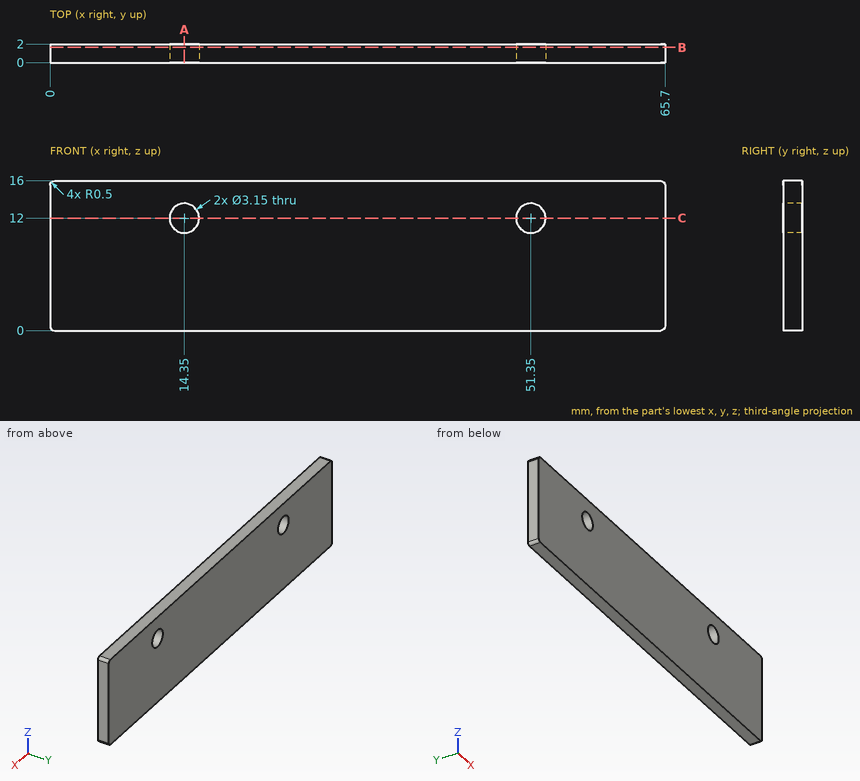
Can you work these out from the drawing? Everything is in mm from the part's minimum corner. Give positions to 0.01 mm unless a question says otherwise; leave off trailing zeros. Loops run counter-clockwise (first coordinate to the right, second up) from the corner with the lowest first, then second, coordinate; pieces in that order, holes last. Notation, with made-up numbers: M 8,-37.5 L 34,-37.5 A28 ccw 34,-8.5 Z; hole C -6.75,-6.5 d11. An arc over 180 degrees is marked long. Use CSV: the item, a comma, the result in double quotes. Start each with the question number.
1. If I drill on L1, parallel to X at y = 1.25, z = 12 (3 decimals); L2, parallel to Z at x = 51.35, y = 0.95 (3 decimals); L3, parallel to Z at x = 51, y = 0.1, over which ranges is the centre line in solid material (lowest first)?
2. Imagine slicing it at A-A, the plane x = 14.35. Write out the boundary of the cut face in (y, z) (3 decimals), plus the area to 3 significant figures.
3. Imagine slicing it at C-C, the plane z = 12. Write out the boundary of the cut face in (x, y) (3 decimals), plus the area to 3 significant figures.
4. For P1, Ø1.9, axis at x = 51.35, z = 12, coming from the +Y side, with a flat end and sliding along its axis, tell me the tip position at first contact or that it passes through.
5. Imagine slicing it at B-B, the plane y = 1.65. Write out the boundary of the cut face in (x, z) (3 decimals).
Response values:
1,L1,"0 to 12.775, 15.925 to 49.775, 52.925 to 65.7"
1,L2,"0 to 10.425, 13.575 to 16"
1,L3,"0 to 10.46, 13.54 to 16"
2,outline,"M 0,0 L 2,0 L 2,10.425 L 0,10.425 Z; M 0,13.575 L 2,13.575 L 2,16 L 0,16 Z"
2,area,"25.7 mm^2"
3,outline,"M 0,0 L 12.775,0 L 12.775,2 L 0,2 Z; M 15.925,0 L 49.775,0 L 49.775,2 L 15.925,2 Z; M 52.925,0 L 65.7,0 L 65.7,2 L 52.925,2 Z"
3,area,"119 mm^2"
4,P1,"through"
5,outline,"M 0,0.5 A0.5 ccw 0.5,0 L 65.2,0 A0.5 ccw 65.7,0.5 L 65.7,15.5 A0.5 ccw 65.2,16 L 0.5,16 A0.5 ccw 0,15.5 Z; hole C 14.35,12 d3.15; hole C 51.35,12 d3.15"
